```python
from build123d import *

# Parameters (mm, degrees)
ESQUISSE1_W             = 400
ESQUISSE1_H             = 80
BOSS_EXTRU_1_DEPTH      = 8
ESQUISSE2_W             = 8
ESQUISSE2_H             = 20
BOSS_EXTRU_2_DEPTH      = 8
ESQUISSE4_W             = 15
ESQUISSE4_H             = 8
ENL_V_MAT_EXTRU_1_DEPTH = 212.962260792
ESQUISSE5_W             = 15
ESQUISSE5_H             = 8
ESQUISSE5_W_2           = 35
ENL_V_MAT_EXTRU_2_DEPTH = 212.962260792
ESQUISSE6_W             = 20
ESQUISSE6_H             = 8
ENL_V_MAT_EXTRU_3_DEPTH = 212.962260792


with BuildPart() as part:
    # Esquisse1 → Boss.-Extru.1 (new body)
    with BuildSketch(Plane.XY):
        Rectangle(ESQUISSE1_W, ESQUISSE1_H)
    extrude(amount=BOSS_EXTRU_1_DEPTH)

    # Esquisse2 → Boss.-Extru.2 (add)
    with BuildSketch(Plane.XY):
        with Locations((-204, 20)):
            Rectangle(ESQUISSE2_W, ESQUISSE2_H)
        with Locations((-204, -20)):
            Rectangle(ESQUISSE2_W, ESQUISSE2_H)
    extrude(amount=BOSS_EXTRU_2_DEPTH)

    # Esquisse4 → Enlèv. mat.-Extru.1 (cut, through all)
    with BuildSketch(Plane.XY):
        Polygon((0, 40), (-15, 40), (-15, 32), (0, 32), (15, 32), (15, 40), align=None)
        with Locations((-37.5, 36)):
            Rectangle(ESQUISSE4_W, ESQUISSE4_H)
        with Locations((-67.5, 36)):
            Rectangle(ESQUISSE4_W, ESQUISSE4_H)
        with Locations((-97.5, 36)):
            Rectangle(ESQUISSE4_W, ESQUISSE4_H)
        with Locations((-127.5, 36)):
            Rectangle(ESQUISSE4_W, ESQUISSE4_H)
        with Locations((-157.5, 36)):
            Rectangle(ESQUISSE4_W, ESQUISSE4_H)
        with Locations((37.5, 36)):
            Rectangle(ESQUISSE4_W, ESQUISSE4_H)
        with Locations((67.5, 36)):
            Rectangle(ESQUISSE4_W, ESQUISSE4_H)
        with Locations((97.5, 36)):
            Rectangle(ESQUISSE4_W, ESQUISSE4_H)
        with Locations((127.5, 36)):
            Rectangle(ESQUISSE4_W, ESQUISSE4_H)
        with Locations((157.5, 36)):
            Rectangle(ESQUISSE4_W, ESQUISSE4_H)
    extrude(amount=ENL_V_MAT_EXTRU_1_DEPTH, mode=Mode.SUBTRACT)

    # Esquisse5 → Enlèv. mat.-Extru.2 (cut, through all)
    with BuildSketch(Plane.XY):
        with Locations((-22.5, -36)):
            Rectangle(ESQUISSE5_W, ESQUISSE5_H)
        with Locations((-52.5, -36)):
            Rectangle(ESQUISSE5_W, ESQUISSE5_H)
        with Locations((-82.5, -36)):
            Rectangle(ESQUISSE5_W, ESQUISSE5_H)
        with Locations((-112.5, -36)):
            Rectangle(ESQUISSE5_W, ESQUISSE5_H)
        with Locations((-142.5, -36)):
            Rectangle(ESQUISSE5_W, ESQUISSE5_H)
        with Locations((-182.5, -36)):
            Rectangle(ESQUISSE5_W_2, ESQUISSE5_H)
        with Locations((22.5, -36)):
            Rectangle(ESQUISSE5_W, ESQUISSE5_H)
        with Locations((52.5, -36)):
            Rectangle(ESQUISSE5_W, ESQUISSE5_H)
        with Locations((82.5, -36)):
            Rectangle(ESQUISSE5_W, ESQUISSE5_H)
        with Locations((112.5, -36)):
            Rectangle(ESQUISSE5_W, ESQUISSE5_H)
        with Locations((142.5, -36)):
            Rectangle(ESQUISSE5_W, ESQUISSE5_H)
        with Locations((182.5, -36)):
            Rectangle(ESQUISSE5_W_2, ESQUISSE5_H)
    extrude(amount=ENL_V_MAT_EXTRU_2_DEPTH, mode=Mode.SUBTRACT)

    # Esquisse6 → Enlèv. mat.-Extru.3 (cut, through all)
    with BuildSketch(Plane.XY):
        with Locations((-160, 0)):
            Rectangle(ESQUISSE6_W, ESQUISSE6_H)
        with Locations((-110, 0)):
            Rectangle(ESQUISSE6_W, ESQUISSE6_H)
    extrude(amount=ENL_V_MAT_EXTRU_3_DEPTH, mode=Mode.SUBTRACT)


solid = part.part
```
Can you work these out from the model? Positions are in its coordinate system, mm. A direction names the side the tool comes from. Give positions to 0.01 mm unless a question says otherwise; leave off trailing zeros. Order: outer loops, then holes, each group sorted by start corner. A loop starts at its lowest first (then second) coordinate and runs counter-clockwise, first axis right, second up. Notation, with made-up numbers: M 27,-21.5 L 37,-21.5 A16 cw 37,-15.5 Z; hole C 3,-15.5 d6. An arc over 180 degrees is marked long. Write item = value, one per line. Start each with the question number.
Q1. Suppose I cut it at B-B (z = 3.25). Count the separate pieces of the cut face and the enclosed holes in it, plus the area to 3 significant figures.
Q2. I need wall thicknesses on probe 1 along X at (y, z) = (-2.5, 5.75); probe 2 along X at (y, z) = (7, 1); probe 3 along Y at (x, z) = (148, 2.5). Which ranges of each line are inside material? Lowest first, please. Write a range as [from, to].
Q3. For faces 1 (the flat face through (-165, -36, 4)), 2 (the flat face through (-120, 36, 4)), 3 (the flat face through (22, -32, 4)), which set-ups out of +Z, -Z, +X, -X, +Y, -Y let a thin tool reach every point of the face, with its end or its side?
Q4. Will these pins go through, and if not, where does the flat tip stop? pin 1 Ø4 at (x, z) = (141.5, 5) entering from -Y; pin 2 Ø4 at (y, z) = (37, 4.5) entering from -X; pin 3 Ø4 at (y, z) = (-35.5, 4) entering from -X.
Q5. Suppose I cut it at A-A (x = -85). Write out the boundary of the cut face in (y, z), plus the area to 3 significant figures.
Q6. We'd pull the mould along X, two halves only. Please class faces 4 (the flat face through (-208, -20, 4)), 5 (the flat face through (200, 3, 4)), 6 (the flat face through (-83, -32, 4)): pulls with the +X half, pulls with the -X half, needs draft (parallel to the pull), parting line crosses it, or undercut.
Check result:
q1.separate_pieces = 1
q1.enclosed_holes = 2
q1.area = 28,800 mm2
q2.probe_1 = [-200, -170], [-150, -120], [-100, 200]
q2.probe_2 = [-200, 200]
q2.probe_3 = [-32, 40]
q3.face_1 = +Z, -Z, -X, -Y
q3.face_2 = +Z, -Z, +Y
q3.face_3 = +Z, -Z, -Y
q4.pin_1 = -32
q4.pin_2 = -200
q4.pin_3 = -165
q5.outline = M -32,0 L 40,0 L 40,8 L -32,8 Z
q5.area = 576 mm2
q6.face_4 = pulls with the -X half
q6.face_5 = pulls with the +X half
q6.face_6 = undercut
